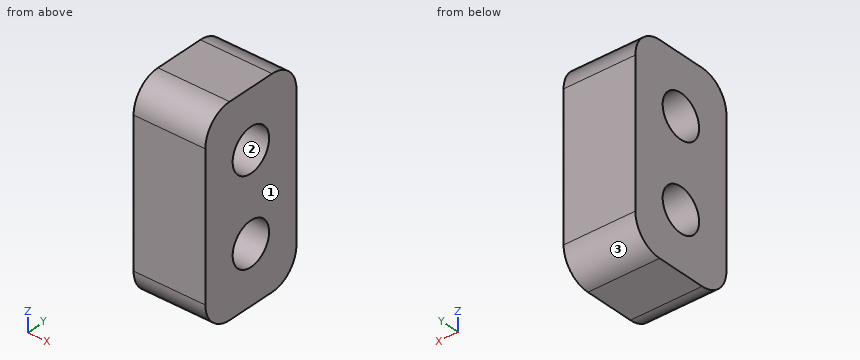
```python
from build123d import *

# Parameters (mm, degrees)
SKETCH1_R           = 1.5
BOSS_EXTRUDE1_DEPTH = 5


with BuildPart() as part:
    # Sketch1 → Boss-Extrude1 (new body)
    with BuildSketch(Plane.YZ):
        with BuildLine():
            Line((0, 2), (0, 12))
            ThreePointArc((0, 12), (0.585786438, 13.414213562), (2, 14))
            Line((2, 14), (5.5, 14))
            ThreePointArc((5.5, 14), (6.914213562, 13.414213562), (7.5, 12))
            Line((7.5, 12), (7.5, 2))
            ThreePointArc((7.5, 2), (6.914213562, 0.585786438), (5.5, 0))
            Line((5.5, 0), (2, 0))
            ThreePointArc((2, 0), (0.585786438, 0.585786438), (0, 2))
        make_face()
        with Locations(Location((3.75, 10, 0), (0, 0, 270))):
            Circle(SKETCH1_R, mode=Mode.SUBTRACT)
        with Locations(Location((3.75, 4, 0), (0, 0, 270))):
            Circle(SKETCH1_R, mode=Mode.SUBTRACT)
    extrude(amount=BOSS_EXTRUDE1_DEPTH)


solid = part.part
```
Can you work these out from the model? Positions are in its coordinate system, mm. Face numbers are marked on the shaded views. Give positions to 0.01 mm unless a question says otherwise; leave off trailing zeros. Write each loop counter-clockwise with the first axis right and the second up, starting at its lowest first coordinate (ties: lowest second). Pieces come first, ordered by that corner, then holes. Notation, with made-up numbers: (19.5, -13.5) -> (66.5, -13.5) arc R11 ccw to (66.5, -6.5) -> close; hole circle Ø4 at (-7.5, 63.5). An arc over 180 degrees is marked (long way). Write item = value, one per line.
(1) Suppose I cut it at A-A on y = 3.75. Write out the boundary of the cut face in (x, z), then the cut area to 3 significant figures.
Worked out:
outline = (0, 0) -> (5, 0) -> (5, 2.5) -> (0, 2.5) -> close; (0, 5.5) -> (5, 5.5) -> (5, 8.5) -> (0, 8.5) -> close; (0, 11.5) -> (5, 11.5) -> (5, 14) -> (0, 14) -> close
area = 40.0 mm^2
(2) Suppose I cut it at C-C on x = 4. Write out the boundary of the cut face in (y, z).
Worked out:
outline = (0, 2) arc R2 ccw to (2, 0) -> (5.5, 0) arc R2 ccw to (7.5, 2) -> (7.5, 12) arc R2 ccw to (5.5, 14) -> (2, 14) arc R2 ccw to (0, 12) -> close; hole circle Ø3 at (3.75, 4); hole circle Ø3 at (3.75, 10)
(3) Suppose I cut it at D-D on z = 4.75. Write out the boundary of the cut face in (x, y).
Worked out:
outline = (0, 0) -> (5, 0) -> (5, 2.45) -> (0, 2.45) -> close; (0, 5.05) -> (5, 5.05) -> (5, 7.5) -> (0, 7.5) -> close
(4) Thinking about a two-plate mould opening in Y: for the marked faces 1, 2 and 3, which applies, released by +Y, released by -Y, zero draft, split by the parting line, or undercut?
Worked out:
face_1 = zero draft
face_2 = undercut
face_3 = released by +Y
(5) Suppose I cut it at B-B on z = 10. Write out the boundary of the cut face in (x, y).
Worked out:
outline = (0, 0) -> (5, 0) -> (5, 2.25) -> (0, 2.25) -> close; (0, 5.25) -> (5, 5.25) -> (5, 7.5) -> (0, 7.5) -> close
(6) I need wall thicknesses on probe 1 along Y at (x, z) = (3.1, 4); probe 2 along Z at (x, y) = (1.3, 4.5); probe 3 along Z at (x, y) = (1.9, 3.5). Which ranges of each line are inside material? Lowest first, please. Write a range as from..to.
Worked out:
probe_1 = 0..2.25, 5.25..7.5
probe_2 = 0..2.7, 5.3..8.7, 11.3..14
probe_3 = 0..2.52, 5.48..8.52, 11.48..14
(7) I'm going to push a flat-ended pin straight in: P1, Ø2, axis at x = 3.5, y = 1.5, coming from the +Z side. Where does the tip first touch, or does it pass through?
Worked out:
P1 = 14
